Input: part model. Units: mm. Frame: model coordinates. A direction names the side the tool comes from. Round coordinates to 2 decimals unless told otherwise and drop trailing zeros. Loops run counter-clockwise (first coordinate to the right, second up) from the corner with the lowest first, then second, coordinate; pieces in that order, holes last. Notation, with made-up numbers: (8, -32) -> (34, -32) arc R24 cw to (34, -7) -> close; hole circle Ø3 at (13, 70). An arc over 180 degrees is marked (long way). One line per question, with ' | ' between items. Start each with the question number.
Q1. Contact query for flat-ended pins moving along their axis: P1, Ø1, axis at y = -2, z = 31.5, coming from the -X side; P2, Ø1, axis at y = -1.5, z = -26, coming from the +X side. Output: stop coordinate, or through.
Q2. Cut plane B-B on y = -0.9. Return loops of the section in (x, z) (1 decimal).
Q3. Material intervals for L1, parallel to X at y = -2.7, z = 79; L2, parallel to X at y = -2.7, z = -72.5; L3, parallel to Z at x = -23.5, y = -1.7, sorted ascending.
Q4. Access query for faces 1 (the face through (17.565, -1.565, 91.459)), 2 (the face through (17.08, -1.57, -91.74)), 3 (the face through (-1, 0, 1)). Directions: +Z, -Z, +X, -X, +Y, -Y. A direction counts if a zero-diameter tool reaches every point of the face in a straight line with its end or side. Return the directions, or none.
Q5. Cut plane C-C on z = 76.2. Return loops of the section in (x, y) (3 decimals).
Q6. Cut plane A-A on z = 0. Return loops of the section in (x, y) (3 decimals), and give its area (3 significant figures).
Q7. Cut plane D-D on x = -68.5. Return loops of the section in (y, z) (1 decimal).
Q8. Mould query, pull axis X, two halves, no side actions, for faces 4 (the face through (70.423, -1.565, -60.941)), 5 (the face through (49.596, -1.565, 85.428)), 6 (the face through (49.18, -1.57, -85.67)), 7 (the face through (-70.91, -1.57, -60.66)). Classes: pulls with the +X half, pulls with the -X half, needs draft (parallel to the pull), parting line crosses it, or undercut.
from build123d import *

# Parameters (mm, degrees)
F1_DEPTH = 3.175
F4_DEPTH = 3.175
F5_R     = 4.445
F6_DEPTH = 3.176


# Not quite as in the source:
# - a length typed as a fraction of an inch, garbled in the dataset ("3 / 203.2 mm" for 3/8 in), is restored


with BuildPart() as f1:
    # F0 (on Front) → F1 (new body)
    with BuildSketch(Plane.XZ):
        Polygon((87.9881810245, 50.8), (0, 101.6), (-87.9881810245, 50.8), (-87.9881810245, -50.8), (0, -101.6), (87.9881810245, -50.8), align=None)
    extrude(amount=F1_DEPTH)

    # F3 (on Front) → F4 (join)
    with BuildSketch(Plane.XZ):
        with BuildLine():
            ThreePointArc((87.9881810245, -10.795), (98.7831810245, 0), (87.9881810245, 10.795))
            Line((87.9881810245, 10.795), (87.9881810245, -10.795))
        make_face()
        with BuildLine():
            Line((34.6453462784, 81.5975), (53.3428347461, 70.8025))
            ThreePointArc((53.3428347461, 70.8025), (49.3915905122, 85.5487442339), (34.6453462784, 81.5975))
        make_face()
        with BuildLine():
            Line((-53.3428347461, 70.8025), (-34.6453462784, 81.5975))
            ThreePointArc((-34.6453462784, 81.5975), (-49.3915905122, 85.5487442339), (-53.3428347461, 70.8025))
        make_face()
        with BuildLine():
            Line((-87.9881810245, -10.795), (-87.9881810245, 10.795))
            ThreePointArc((-87.9881810245, 10.795), (-98.7831810245, 0), (-87.9881810245, -10.795))
        make_face()
        with BuildLine():
            Line((-34.6453462784, -81.5975), (-53.3428347461, -70.8025))
            ThreePointArc((-53.3428347461, -70.8025), (-49.3915905122, -85.5487442339), (-34.6453462784, -81.5975))
        make_face()
        with BuildLine():
            Line((53.3428347461, -70.8025), (34.6453462784, -81.5975))
            ThreePointArc((34.6453462784, -81.5975), (49.3915905122, -85.5487442339), (53.3428347461, -70.8025))
        make_face()
    extrude(amount=F4_DEPTH)

    # F5 (on face) → F6 (cut, through all)
    with BuildSketch(Plane.XZ.offset(3.175)):
        with Locations((43.9940905122, 76.2)):
            Circle(F5_R)
        with Locations((-43.9940905122, 76.2)):
            Circle(F5_R)
        with Locations((-87.9881810245, 0)):
            Circle(F5_R)
        with Locations((-43.9940905122, -76.2)):
            Circle(F5_R)
        with Locations((43.9940905122, -76.2)):
            Circle(F5_R)
        with Locations((87.9881810245, 0)):
            Circle(F5_R)
    extrude(amount=-F6_DEPTH, mode=Mode.SUBTRACT)


solid = f1.part
Results:
1) P1: x = -87.99 | P2: x = 87.99
2) outline: (-88, -50.8) -> (-53.3, -70.8) arc R10.8 ccw to (-34.6, -81.6) -> (0, -101.6) -> (34.6, -81.6) arc R10.8 ccw to (53.3, -70.8) -> (88, -50.8) -> (88, -10.8) arc R10.8 ccw to (88, 10.8) -> (88, 50.8) -> (53.3, 70.8) arc R10.8 ccw to (34.6, 81.6) -> (0, 101.6) -> (-34.6, 81.6) arc R10.8 ccw to (-53.3, 70.8) -> (-88, 50.8) -> (-88, 10.8) arc R10.8 ccw to (-88, -10.8) -> close; hole circle Ø8.9 at (-88, 0); hole circle Ø8.9 at (-44, -76.2); hole circle Ø8.9 at (-44, 76.2); hole circle Ø8.9 at (44, -76.2); hole circle Ø8.9 at (44, 76.2); hole circle Ø8.9 at (88, 0)
3) L1: -54.42 to -47.45, -40.54 to 40.54, 47.45 to 54.42 | L2: -54.14 to -46.46, -41.53 to 41.53, 46.46 to 54.14 | L3: -88.03 to 88.03
4) face 1: +Z, +Y, -Y | face 2: -Z, +Y, -Y | face 3: +Z, -Z, +X, -X, +Y
5) outline: (-54.789, -3.175) -> (-48.439, -3.175) -> (-48.439, 0) -> (-54.789, 0) -> close; (-39.549, -3.175) -> (39.549, -3.175) -> (39.549, 0) -> (-39.549, 0) -> close; (48.439, -3.175) -> (54.789, -3.175) -> (54.789, 0) -> (48.439, 0) -> close
6) outline: (-98.783, -3.175) -> (-92.433, -3.175) -> (-92.433, 0) -> (-98.783, 0) -> close; (-83.543, -3.175) -> (83.543, -3.175) -> (83.543, 0) -> (-83.543, 0) -> close; (92.433, -3.175) -> (98.783, -3.175) -> (98.783, 0) -> (92.433, 0) -> close | area: 571 mm^2
7) outline: (-3.2, -62.1) -> (0, -62.1) -> (0, 62.1) -> (-3.2, 62.1) -> close
8) face 4: pulls with the +X half | face 5: undercut | face 6: undercut | face 7: pulls with the -X half
